The listing builds one solid part. Answer for the finished solid, in the listing's coordinates (mm). A direction names the side the tool comes from. Give positions to 0.01 mm unless a question says otherwise; leave off trailing zeros. Loops run counter-clockwise (first coordinate to the right, second up) from the corner with the lowest first, then second, coordinate; pieces in that order, holes last.
Item 1: Section A-A, the plane z = 368.3 is taken. Give the vertices of the cut face in (x, y) (3 decimals).
Item 2: Section C-C, the plane z = 132 is taken. Give the vertices of the cut face in (x, y) (3 decimals).
Item 3: Section B-B, the plane y = -143.5 is taken. Give the number of separate pieces and of enclosed holes in the cut face, and give its area (3 significant figures).
Item 4: Consider line 1 along X through (y, z) = (-135, 254) (3 decimals); line 2 along Z through (x, y) = (-206.5, -110); line 3 along Y through (x, z) = (-194, 368). Determine where each line is inside the solid, lowest interval first.
Item 5: Each of these flat-tipped pins is pushed along its axis until it touches: pin 1 Ø10 at (x, y) = (320.5, -142) entering from +Z; pin 2 Ø2 at (x, y) = (284, -261.5) entering from -Z; pin 3 Ø11.5 at (y, z) = (-12.7, 368.3) entering from +X. Where does it stop, or does it pass through?
Item 6: The mould has two halves that part along Y. Classify faces 3 (the face through (-381, -170, 234.061)), 4 (the face through (-381, -2.54, 294)), 5 (the face through (-6.71, -330.66, 380.99)), 6 (the face through (-6.71, -329.74, -25.39)): pulls with the +Y half, pulls with the -Y half, needs draft (parallel to the pull), parting line crosses it, or undercut.
Item 7: A tool of negligible diameter and unlimited length cuts with its end or side. For faces 1 (the face through (-190, -2.54, 60)), 2 (the face through (-479.425, -174, 181)), from which of +Z, -Z, +X, -X, +Y, -Y can it reach the whole face along a straight path? Write none if from no direction.
from build123d import *

# Parameters (mm, degrees)
F0_W     = 342.9
F0_H     = 355.6
F1_DEPTH = 479.425
F2_T     = -2.54
F3_R     = 9.525
F4_DEPTH = 958.85
F5_W     = 958.85
F5_H     = 355.6
F5_W_2   = 182.245
F5_H_2   = 109.347
F5_W_3   = 185.42
F5_H_3   = 112.014
F5_H_4   = 108.839
F6_DEPTH = 342.9
F7_R     = 1.016


with BuildPart() as f1:
    # F0 (on Right) → F1 (new body, symmetric)
    with BuildSketch(Plane.YZ):
        with Locations((-171.45, 177.8)):
            Rectangle(F0_W, F0_H)
    extrude(amount=F1_DEPTH, both=True)

    # F2
    f2_openings = [f1.faces().sort_by_distance(p)[0] for p in [
        (0, -342.9, 177.8),
    ]]
    offset(amount=F2_T, openings=f2_openings)

    # F3 (on face) → F4 (join, through all)
    with BuildSketch(Plane(origin=(-479.425, 0, 0), x_dir=(0, -1, 0), z_dir=(-1, 0, 0))):
        with BuildLine():
            Line((19.05, 355.6), (19.05, 357.3014773719))
            ThreePointArc((19.05, 357.3014773719), (12.7, 381), (6.35, 357.3014773719))
            Line((6.35, 357.3014773719), (6.35, 355.6))
            Line((6.35, 355.6), (19.05, 355.6))
        make_face()
        with Locations((12.7, 368.3)):
            Circle(F3_R, mode=Mode.SUBTRACT)
        with BuildLine():
            Line((336.55, 355.6), (336.55, 357.3014773719))
            ThreePointArc((336.55, 357.3014773719), (330.2, 381), (323.85, 357.3014773719))
            Line((323.85, 357.3014773719), (323.85, 355.6))
            Line((323.85, 355.6), (336.55, 355.6))
        make_face()
        with Locations((330.2, 368.3)):
            Circle(F3_R, mode=Mode.SUBTRACT)
        with BuildLine():
            Line((6.35, 0), (6.35, -1.7014773719))
            ThreePointArc((6.35, -1.7014773719), (12.7, -25.4), (19.05, -1.7014773719))
            Line((19.05, -1.7014773719), (19.05, 0))
            Line((19.05, 0), (6.35, 0))
        make_face()
        with Locations((12.7, -12.7)):
            Circle(F3_R, mode=Mode.SUBTRACT)
        with BuildLine():
            Line((323.85, 0), (323.85, -1.7014773719))
            ThreePointArc((323.85, -1.7014773719), (330.2, -25.4), (336.55, -1.7014773719))
            Line((336.55, -1.7014773719), (336.55, 0))
            Line((336.55, 0), (323.85, 0))
        make_face()
        with Locations((330.2, -12.7)):
            Circle(F3_R, mode=Mode.SUBTRACT)
    extrude(amount=-F4_DEPTH)

    # F5 (on face) → F6 (join, through all)
    with BuildSketch(Plane(origin=(0, 0, 0), x_dir=(-1, 0, 0), z_dir=(0, 1, 0))):
        with Locations((0, 177.8)):
            Rectangle(F5_W, F5_H)
        with Locations((-381.9525, 61.0235)):
            Rectangle(F5_W_2, F5_H_2, mode=Mode.SUBTRACT)
        with Locations((-191.77, 61.0235)):
            Rectangle(F5_W_3, F5_H_2, mode=Mode.SUBTRACT)
        with Locations((0, 61.0235)):
            Rectangle(F5_W_3, F5_H_2, mode=Mode.SUBTRACT)
        with Locations((191.77, 61.0235)):
            Rectangle(F5_W_3, F5_H_2, mode=Mode.SUBTRACT)
        with Locations((381.9525, 61.0235)):
            Rectangle(F5_W_2, F5_H_2, mode=Mode.SUBTRACT)
        with Locations((-381.9525, 178.054)):
            Rectangle(F5_W_2, F5_H_3, mode=Mode.SUBTRACT)
        with Locations((-191.77, 178.054)):
            Rectangle(F5_W_3, F5_H_3, mode=Mode.SUBTRACT)
        with Locations((0, 178.054)):
            Rectangle(F5_W_3, F5_H_3, mode=Mode.SUBTRACT)
        with Locations((-381.9525, 294.8305)):
            Rectangle(F5_W_2, F5_H_4, mode=Mode.SUBTRACT)
        with Locations((-191.77, 294.8305)):
            Rectangle(F5_W_3, F5_H_4, mode=Mode.SUBTRACT)
        with Locations((0, 294.8305)):
            Rectangle(F5_W_3, F5_H_4, mode=Mode.SUBTRACT)
        with Locations((191.77, 178.054)):
            Rectangle(F5_W_3, F5_H_3, mode=Mode.SUBTRACT)
        with Locations((381.9525, 178.054)):
            Rectangle(F5_W_2, F5_H_3, mode=Mode.SUBTRACT)
        with Locations((191.77, 294.8305)):
            Rectangle(F5_W_3, F5_H_4, mode=Mode.SUBTRACT)
        with Locations((381.9525, 294.8305)):
            Rectangle(F5_W_2, F5_H_4, mode=Mode.SUBTRACT)
    extrude(amount=-F6_DEPTH)

    # F7
    f7_edges = [f1.edges().sort_by_distance(p)[0] for p in [
        (0, -336.55, 357.301477),
        (0, -336.55, 355.6),
        (0, -323.85, 357.301477),
        (0, -323.85, 355.6),
        (0, -19.05, 355.6),
        (0, -19.05, 357.301477),
        (0, -6.35, 357.301477),
        (0, -6.35, 355.6),
        (0, -6.35, 0),
        (0, -6.35, -1.701477),
        (0, -19.05, 0),
        (0, -19.05, -1.701477),
        (0, -323.85, -1.701477),
        (0, -323.85, 0),
        (0, -336.55, 0),
        (0, -336.55, -1.701477),
    ]]
    fillet(f7_edges, radius=F7_R)


solid = f1.part
Worked answers:
1. outline: (-479.425, -342.9) - (479.425, -342.9) - (479.425, -339.725) - (-479.425, -339.725) - close; (-479.425, -320.675) - (479.425, -320.675) - (479.425, -317.5) - (-479.425, -317.5) - close; (-479.425, -25.4) - (479.425, -25.4) - (479.425, -22.225) - (-479.425, -22.225) - close; (-479.425, -3.175) - (479.425, -3.175) - (479.425, 0) - (-479.425, 0) - close
2. outline: (-479.425, -342.9) - (-473.075, -342.9) - (-473.075, -2.54) - (-290.83, -2.54) - (-290.83, -342.9) - (-284.48, -342.9) - (-284.48, -2.54) - (-99.06, -2.54) - (-99.06, -342.9) - (-92.71, -342.9) - (-92.71, -2.54) - (92.71, -2.54) - (92.71, -342.9) - (99.06, -342.9) - (99.06, -2.54) - (284.48, -2.54) - (284.48, -342.9) - (290.83, -342.9) - (290.83, -2.54) - (473.075, -2.54) - (473.075, -342.9) - (479.425, -342.9) - (479.425, 0) - (-479.425, 0) - close
3. separate pieces: 1
3. enclosed holes: 15
3. area: 36,900 mm2
4. line 1: x = -479.425 to -473.075, -290.83 to -284.48, -99.06 to -92.71, 92.71 to 99.06, 284.48 to 290.83, 473.075 to 479.425
4. line 2: z = 0 to 6.35, 115.7 to 122.05, 234.06 to 240.41, 349.25 to 355.6
4. line 3: y = -342.9 to -339.72, -320.68 to -317.5, -25.4 to -22.22, -3.18 to 0
5. pin 1: stops at z = 355.6
5. pin 2: stops at z = 0
5. pin 3: passes through
6. face 3: needs draft
6. face 4: pulls with the -Y half
6. face 5: undercut
6. face 6: undercut
7. face 1: -Y
7. face 2: +Z, -Z, -X, +Y, -Y
